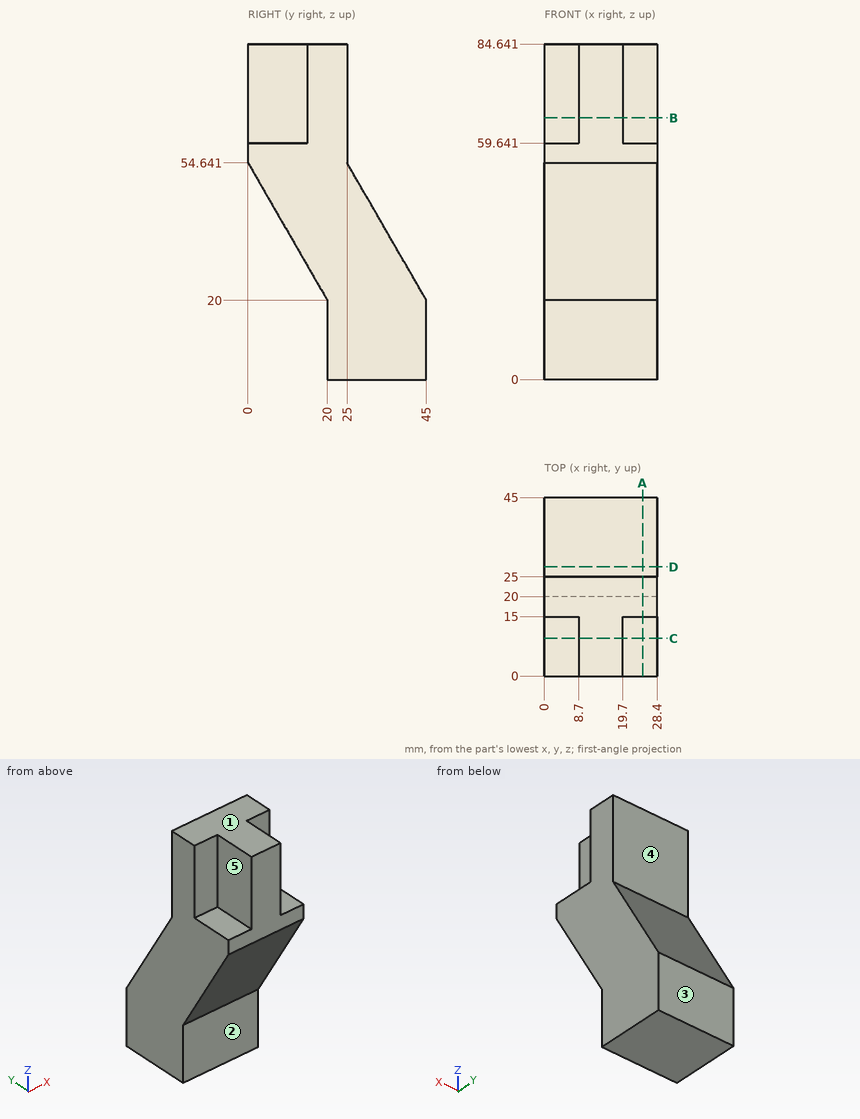
Answer from the drawing. Dimensions are ordinates in mm from the lowest x, y and z of the part. A direction names the side the tool comes from. Round coordinates to 2 decimals unless told otherwise and drop trailing zeros. Order: outer loops, then holes, each group sorted by start corner. A loop starts at its lowest first (then second) coordinate and runs counter-clockwise, first axis right, second up.
1) The part is cut by section D-D on y = 27.5. Write down the section's boundary in (x, z).
2) Straight lines are drawn through the part: L1, parallel to Y at x = 8, z = 74; L2, parallel to Y at x = 14.5, z = 19.5; L3, parallel to Z at x = 14, y = 7. For each, find the intervals that lie inside material, in ascending order.
3) The part is cut by section B-B on z = 66. Write down the section's boundary in (x, y), plus the area to 3 significant figures.
4) The part is cut by section C-C on y = 9.5. Write down the section's boundary in (x, z).
5) For the marked faces 1, 2, 3, 4 and 5, determine the directions among +Z, -Z, +X, -X, +Y, -Y from which every point of the face is accessible in a straight line to the end or side of a thin tool.
6) The part is cut by section A-A on x = 24.75. Write down the section's boundary in (y, z), plus the area to 3 significant figures.
7) Flat-ended cylindrical pins translate along their axes: pin 1 (8.5 mm diameter, centred on x = 15, z = 71, fed in from +Y); pin 2 (10 mm diameter, centred on x = 8.5, z = 5.5, fed in from -Y); pin 3 (2.5 mm diameter, centred on x = 22.5, y = 5, fed in from +Z). Find the tip coordinate at first contact, or state that the pin passes through.
Resolved:
1. outline: (0, 0) - (28.4, 0) - (28.4, 50.31) - (0, 50.31) - close
2. L1: y = 15 to 25
2. L2: y = 20 to 45
2. L3: z = 42.52 to 84.64
3. outline: (0, 15) - (8.7, 15) - (8.7, 0) - (19.7, 0) - (19.7, 15) - (28.4, 15) - (28.4, 25) - (0, 25) - close
3. area: 449 mm2
4. outline: (0, 38.19) - (28.4, 38.19) - (28.4, 59.64) - (19.7, 59.64) - (19.7, 84.64) - (8.7, 84.64) - (8.7, 59.64) - (0, 59.64) - close
5. face 1: +Z, +X, -X, +Y, -Y
5. face 2: -Z, +X, -X, -Y
5. face 3: +Z, -Z, +X, -X, +Y
5. face 4: +Z, +X, -X, +Y
5. face 5: +Z, -X, -Y
6. outline: (0, 54.64) - (20, 20) - (20, 0) - (45, 0) - (45, 20) - (25, 54.64) - (25, 84.64) - (15, 84.64) - (15, 59.64) - (0, 59.64) - close
6. area: 1,740 mm2
7. pin 1: stops at y = 25
7. pin 2: stops at y = 20
7. pin 3: stops at z = 59.64
